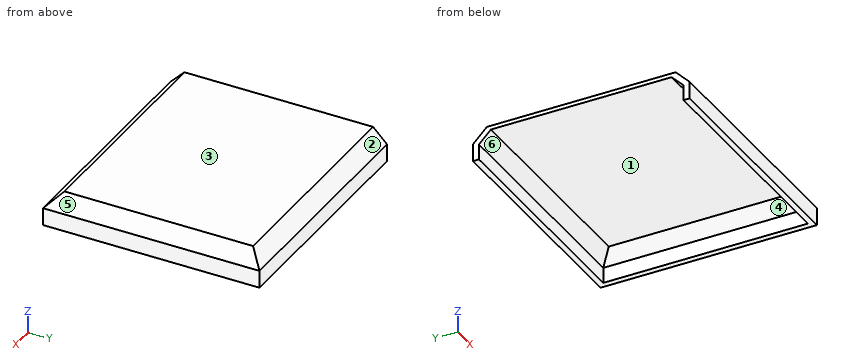
```python
from build123d import *

# Parameters (mm, degrees)
BOX035_W               = 117
BOX035_H               = 104
BOX035_DEPTH           = 14
CHAMFER004_SIZE        = 6.07
BOX034_W               = 120
BOX034_H               = 110
BOX034_DEPTH           = 16
CHAMFER003_SIZE        = 7.07
CUT032_PLACEMENT_ANGLE = 180


with BuildPart() as chamfer004:
    # Box035 → Box035 (new body)
    with BuildSketch(Plane(origin=(0, 3, 2), x_dir=(1, 0, 0), z_dir=(0, 0, 1))):
        with Locations((58.5, 52)):
            Rectangle(BOX035_W, BOX035_H)
    extrude(amount=BOX035_DEPTH)

    # Chamfer004
    chamfer004_edges = [chamfer004.edges().sort_by_distance(p)[0] for p in [
        (117, 55, 2),
        (58.5, 3, 2),
        (58.5, 107, 2),
    ]]
    chamfer(chamfer004_edges, length=CHAMFER004_SIZE)


with BuildPart() as deckel_cut_basis:
    # Box034 → Box034 (new body)
    with BuildSketch(Plane.XY):
        with Locations((60, 55)):
            Rectangle(BOX034_W, BOX034_H)
    extrude(amount=BOX034_DEPTH)

    # Chamfer003
    chamfer003_edges = [deckel_cut_basis.edges().sort_by_distance(p)[0] for p in [
        (120, 55, 0),
        (60, 0, 0),
        (60, 110, 0),
    ]]
    chamfer(chamfer003_edges, length=CHAMFER003_SIZE)

    # Cut032: cut Chamfer004
    add(chamfer004.part, mode=Mode.SUBTRACT)


with BuildPart() as deckel_cut_basis_1:
    # Cut032 placement: moved
    add(deckel_cut_basis.part.rotate(Axis((0, 0, 0), (1, 0, 0)), CUT032_PLACEMENT_ANGLE))


with BuildPart() as obj1:
    # mirror: instance of Deckel_Cut_Basis
    add(deckel_cut_basis_1.part.mirror(Plane(origin=(0, 0, 0), x_dir=(1, 0, 0), z_dir=(0, 1, 0))))


with BuildPart() as obj1_1:
    # mirror placement: moved
    add(obj1.part.moved(Location((0, 0, 16))))


solid = obj1_1.part
```
Verification items for the finished model (mm, model axes). Face numbers are marked on the shaded views. A direction names the side the tool comes from. Give positions to 0.01 mm unless a question says otherwise; leave off trailing zeros. Loops run counter-clockwise (first coordinate to the right, second up) from the corner with the lowest first, then second, coordinate; pieces in that order, holes last.
1. Section check B-B, the plane z = 10.5. Enter the section's corners in (x, y), then the cut area to 3 significant figures.
2. Section check A-A, the plane x = 78. Enter the section's corners in (y, z).
3. Thickness scan on line 1 (Y direction, x = 92.5, z = 1.75); line 2 (Z direction, x = 93, y = 63.5); line 3 (X direction, y = 86.5, z = 0.5). Record the ranges inside material, lowest first.
4. Go/stop test with flat-tipped pins: pin 1 Ø1.5 at (x, z) = (69, 13) entering from -Y; pin 2 Ø6.5 at (y, z) = (80.5, 3.5) entering from -X; pin 3 Ø1 at (x, y) = (85.5, 28.5) entering from -Z. Record where each tip stops, or that it passes through.
5. Mould release check, pull along Y, two halves, no side actions. Record for the marked faces 1, 2, 3 and 4: released by +Y, released by -Y, zero draft, split by the parting line, or undercut.
6. Section check C-C, the plane y = 59. Enter the section's corners in (x, z).
7. Set-up check for the marked faces 5 and 6: record each of +Z, -Z, +X, -X, +Y, -Y from which the full face is reachable in a straight line by a thin tool's end or side.
Geometry says:
1. outline: (0, 1.57) - (118.43, 1.57) - (118.43, 108.43) - (0, 108.43) - (0, 104.43) - (114.43, 104.43) - (114.43, 5.57) - (0, 5.57) - close
1. area: 1,340 mm2
2. outline: (0, 0) - (3, 0) - (3, 7.93) - (9.07, 14) - (100.93, 14) - (107, 7.93) - (107, 0) - (110, 0) - (110, 8.93) - (102.93, 16) - (7.07, 16) - (0, 8.93) - close
3. line 1: y = 0 to 3, 107 to 110
3. line 2: z = 14 to 16
3. line 3: x = 117 to 120
4. pin 1: stops at y = 3.32
4. pin 2: stops at x = 117
4. pin 3: stops at z = 14
5. face 1: undercut
5. face 2: released by +Y
5. face 3: zero draft
5. face 4: undercut
6. outline: (0, 14) - (110.93, 14) - (117, 7.93) - (117, 0) - (120, 0) - (120, 8.93) - (112.93, 16) - (0, 16) - close
7. face 5: +Z, +X, +Y, -Y
7. face 6: -Z, -X
